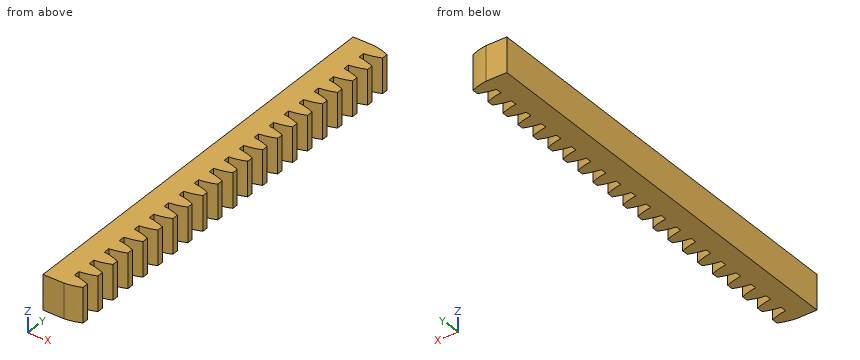
Autodesk Inventor part; units mm, degrees
ref_plane "YZ Plane" through (0, 0, 0) normal (1, 0, 0) x (0, 1, 0)
ref_plane "XZ Plane" through (0, 0, 0) normal (0, 1, 0) x (-1, 0, 0)
ref_plane "XY Plane" through (0, 0, 0) normal (0, 0, 1) x (1, 0, 0)
ref_plane "Arbeitsebene1" through (0, 0, -5) normal (0, 0, -1) x (-1, 0, 0)
sketch "Skizze1" plane through (0, 0, -5) normal (0, 0, -1) x (-1, 0, 0)
  arc A0 (8.6893, -1.0285) -> (10.9915, -0.4319) centre (7.7825, 7.211) ccw
  arc A1 (10.9915, -0.4319) -> (10.9915, 0.4319) centre (0, 0) ccw
  arc A2 (10.9915, 0.4319) -> (8.6893, 1.0285) centre (7.7825, -7.211) ccw
  line L0 (8.6893, -1.0285) -> (8.6893, 1.0285) construction
  arc A3 (12.6615, 1.2584) -> (14.9637, 0.6618) centre (15.8705, 8.9013) ccw
  arc A4 (12.6615, 2.1221) -> (12.6615, 1.2584) centre (23.6531, 1.6903) ccw
  arc A5 (14.9637, 2.7187) -> (12.6615, 2.1221) centre (15.8705, -5.5208) ccw
  arc A6 (8.6893, 1.0285) -> (8.5819, 1.707) centre (0, 0) ccw construction
  arc A7 (8.6893, 1.0285) -> (8.5819, 1.707) centre (0, 0) ccw construction
  arc A8 (8.6893, 1.0285) -> (8.5819, 1.707) centre (0, 0) ccw construction
  arc A9 (8.6893, 1.0285) -> (8.5819, 1.707) centre (0, 0) ccw construction
  arc A10 (8.6893, 1.0285) -> (8.5819, 1.707) centre (0, 0) ccw construction
  arc A11 (12.6615, 4.1794) -> (14.9637, 3.5828) centre (15.8705, 11.8223) ccw
  arc A12 (12.6615, 5.0431) -> (12.6615, 4.1794) centre (23.6531, 4.6113) ccw
  arc A13 (14.9637, 5.6397) -> (12.6615, 5.0431) centre (15.8705, -2.5998) ccw
  arc A14 (12.6615, 7.1004) -> (14.9637, 6.5038) centre (15.8705, 14.7433) ccw
  arc A15 (12.6615, 7.9641) -> (12.6615, 7.1004) centre (23.6531, 7.5323) ccw
  arc A16 (14.9637, 8.5607) -> (12.6615, 7.9641) centre (15.8705, 0.3212) ccw
  arc A17 (12.6615, 10.0214) -> (14.9637, 9.4248) centre (15.8705, 17.6643) ccw
  arc A18 (12.6615, 10.8851) -> (12.6615, 10.0214) centre (23.6531, 10.4533) ccw
  arc A19 (14.9637, 11.4817) -> (12.6615, 10.8851) centre (15.8705, 3.2422) ccw
  arc A20 (12.6615, 12.9424) -> (14.9637, 12.3458) centre (15.8705, 20.5853) ccw
  arc A21 (12.6615, 13.8061) -> (12.6615, 12.9424) centre (23.6531, 13.3743) ccw
  arc A22 (14.9637, 14.4027) -> (12.6615, 13.8061) centre (15.8705, 6.1632) ccw
  arc A23 (12.6615, 15.8634) -> (14.9637, 15.2668) centre (15.8705, 23.5063) ccw
  arc A24 (12.6615, 16.7271) -> (12.6615, 15.8634) centre (23.6531, 16.2953) ccw
  arc A25 (14.9637, 17.3237) -> (12.6615, 16.7271) centre (15.8705, 9.0842) ccw
  arc A26 (12.6615, 18.7844) -> (14.9637, 18.1878) centre (15.8705, 26.4273) ccw
  arc A27 (12.6615, 19.6481) -> (12.6615, 18.7844) centre (23.6531, 19.2163) ccw
  arc A28 (14.9637, 20.2447) -> (12.6615, 19.6481) centre (15.8705, 12.0052) ccw
  arc A29 (12.6615, 21.7054) -> (14.9637, 21.1088) centre (15.8705, 29.3483) ccw
  arc A30 (12.6615, 22.5691) -> (12.6615, 21.7054) centre (23.6531, 22.1373) ccw
  arc A31 (14.9637, 23.1657) -> (12.6615, 22.5691) centre (15.8705, 14.9262) ccw
  arc A32 (12.6615, 24.6264) -> (14.9637, 24.0298) centre (15.8705, 32.2693) ccw
  arc A33 (12.6615, 25.4901) -> (12.6615, 24.6264) centre (23.6531, 25.0583) ccw
  arc A34 (14.9637, 26.0867) -> (12.6615, 25.4901) centre (15.8705, 17.8472) ccw
  arc A35 (12.6615, 27.5474) -> (14.9637, 26.9508) centre (15.8705, 35.1903) ccw
  arc A36 (12.6615, 28.4111) -> (12.6615, 27.5474) centre (23.6531, 27.9793) ccw
  arc A37 (14.9637, 29.0077) -> (12.6615, 28.4111) centre (15.8705, 20.7682) ccw
  arc A38 (12.6615, 30.4684) -> (14.9637, 29.8718) centre (15.8705, 38.1113) ccw
  arc A39 (12.6615, 31.3321) -> (12.6615, 30.4684) centre (23.6531, 30.9003) ccw
  arc A40 (14.9637, 31.9287) -> (12.6615, 31.3321) centre (15.8705, 23.6892) ccw
  arc A41 (12.6615, 33.3894) -> (14.9637, 32.7928) centre (15.8705, 41.0323) ccw
  arc A42 (12.6615, 34.2531) -> (12.6615, 33.3894) centre (23.6531, 33.8213) ccw
  arc A43 (14.9637, 34.8497) -> (12.6615, 34.2531) centre (15.8705, 26.6102) ccw
  arc A44 (12.6615, 36.3104) -> (14.9637, 35.7138) centre (15.8705, 43.9533) ccw
  arc A45 (12.6615, 37.1741) -> (12.6615, 36.3104) centre (23.6531, 36.7423) ccw
  arc A46 (14.9637, 37.7707) -> (12.6615, 37.1741) centre (15.8705, 29.5312) ccw
  arc A47 (12.6615, 39.2314) -> (14.9637, 38.6348) centre (15.8705, 46.8743) ccw
  arc A48 (12.6615, 40.0951) -> (12.6615, 39.2314) centre (23.6531, 39.6633) ccw
  arc A49 (14.9637, 40.6917) -> (12.6615, 40.0951) centre (15.8705, 32.4522) ccw
  arc A50 (12.6615, 42.1524) -> (14.9637, 41.5558) centre (15.8705, 49.7953) ccw
  arc A51 (12.6615, 43.0161) -> (12.6615, 42.1524) centre (23.6531, 42.5843) ccw
  arc A52 (14.9637, 43.6127) -> (12.6615, 43.0161) centre (15.8705, 35.3732) ccw
  arc A53 (12.6615, 45.0734) -> (14.9637, 44.4768) centre (15.8705, 52.7163) ccw
  arc A54 (12.6615, 45.9371) -> (12.6615, 45.0734) centre (23.6531, 45.5053) ccw
  arc A55 (14.9637, 46.5337) -> (12.6615, 45.9371) centre (15.8705, 38.2942) ccw
  arc A56 (12.6615, 47.9944) -> (14.9637, 47.3978) centre (15.8705, 55.6373) ccw
  arc A57 (12.6615, 48.8581) -> (12.6615, 47.9944) centre (23.6531, 48.4263) ccw
  arc A58 (14.9637, 49.4547) -> (12.6615, 48.8581) centre (15.8705, 41.2152) ccw
  arc A59 (12.6615, 50.9154) -> (14.9637, 50.3188) centre (15.8705, 58.5583) ccw
  arc A60 (12.6615, 51.7791) -> (12.6615, 50.9154) centre (23.6531, 51.3473) ccw
  arc A61 (14.9637, 52.3757) -> (12.6615, 51.7791) centre (15.8705, 44.1362) ccw
  arc A62 (12.6615, 53.8364) -> (14.9637, 53.2398) centre (15.8705, 61.4793) ccw
  arc A63 (12.6615, 54.7001) -> (12.6615, 53.8364) centre (23.6531, 54.2683) ccw
  arc A64 (14.9637, 55.2967) -> (12.6615, 54.7001) centre (15.8705, 47.0572) ccw
  arc A65 (12.6615, 56.7574) -> (14.9637, 56.1608) centre (15.8705, 64.4003) ccw
  arc A66 (12.6615, 57.6211) -> (12.6615, 56.7574) centre (23.6531, 57.1893) ccw
  arc A67 (14.9637, 58.2177) -> (12.6615, 57.6211) centre (15.8705, 49.9782) ccw
  arc A68 (12.6615, 59.6784) -> (14.9637, 59.0818) centre (15.8705, 67.3213) ccw
  arc A69 (12.6615, 60.5421) -> (12.6615, 59.6784) centre (23.6531, 60.1103) ccw
  arc A70 (14.9637, 61.1387) -> (12.6615, 60.5421) centre (15.8705, 52.8992) ccw
  line L1 (14.9637, 61.1387) -> (17.9637, 61.1387)
  line L2 (17.9637, 61.1387) -> (17.9637, 0.6618)
  line L3 (17.9637, 0.6618) -> (14.9637, 0.6618)
  line L4 (14.9637, 2.7187) -> (14.9637, 3.5828)
  line L5 (14.9637, 5.6397) -> (14.9637, 6.5038)
  line L6 (14.9637, 8.5607) -> (14.9637, 9.4248)
  line L7 (14.9637, 11.4817) -> (14.9637, 12.3458)
  line L8 (14.9637, 14.4027) -> (14.9637, 15.2668)
  line L9 (14.9637, 17.3237) -> (14.9637, 18.1878)
  line L10 (14.9637, 20.2447) -> (14.9637, 21.1088)
  line L11 (14.9637, 23.1657) -> (14.9637, 24.0298)
  line L12 (14.9637, 26.0867) -> (14.9637, 26.9508)
  line L13 (14.9637, 29.0077) -> (14.9637, 29.8718)
  line L14 (14.9637, 31.9287) -> (14.9637, 32.7928)
  line L15 (14.9637, 34.8497) -> (14.9637, 35.7138)
  line L16 (14.9637, 37.7707) -> (14.9637, 38.6348)
  line L17 (14.9637, 40.6917) -> (14.9637, 41.5558)
  line L18 (14.9637, 43.6127) -> (14.9637, 44.4768)
  line L19 (14.9637, 46.5337) -> (14.9637, 47.3978)
  line L20 (14.9637, 49.4547) -> (14.9637, 50.3188)
  line L21 (14.9637, 52.3757) -> (14.9637, 53.2398)
  line L22 (14.9637, 55.2967) -> (14.9637, 56.1608)
  line L23 (14.9637, 58.2177) -> (14.9637, 59.0818)
  point P0 (14.9637, 32.3608)
extrude "Extrusion1" add sketch "Skizze1" against normal blind 5
properties part number "Zahnstange"
Check sheet for the modelled part. Datum: model origin and axes. Units: mm. Give positions to 0.01 mm unless a question says otherwise; leave off trailing zeros. Answer as CSV lines item,"result". Start each with the question number.
Item 1: Cross-section at A-A on x = -14.4. State how many separate pieces and enclosed holes the cut face has, plus the area to 3 significant figures.
Item 2: Gauge pin test, flat end, axial feed: P1, Ø0.7, axis at y = 44, z = -3, coming from the +X side. Record the tip position at first contact, or that the pin passes through.
Item 3: Thickness scan on line 1 (X direction, y = 32, z = -2.4); line 2 (X direction, y = 36.5, z = -3). Record the ranges inside material, lowest first. Write a range as [from, to].
Established:
1,separate pieces,"21"
1,enclosed holes,"0"
1,area,"199 mm^2"
2,P1,"stops at x = -14.96"
3,line 1,"x = [-17.96, -14.96]"
3,line 2,"x = [-17.96, -12.66]"
